Model file for the job. Use its own axes, mm. Give positions to 0.01 mm unless a question says otherwise; leave off trailing zeros. Order: outer loops, then holes, each group sorted by start corner. A loop starts at its lowest first (then second) coordinate and runs counter-clockwise, first axis right, second up. Notation, with made-up numbers: M 64,20.5 L 83,20.5 A33 cw 83,54.5 Z; hole C 8,-25 d1. An arc over 180 degrees is marked long. Return JSON: item names as keys, results as strings. Group by question number.
1. Slice it at A-A on z = 4. Give the number of separate pieces and of enclosed holes in the cut face, then the cut area to 3 significant figures.
2. Slice it at B-B on y = 16. List the corners of the cut face in (x, z) (3 decimals).
3. Slice it at D-D on y = -3. List the corners of the cut face in (x, z).
4. Wall check: probe 1 along X at (y, z) = (-8.5, 3.95); probe 2 along Y at (x, z) = (-1, 4.55); probe 3 along Z at (x, y) = (-2.5, 2). Give the ranges that are in metal, low to high. Write a range as [from, to].
from build123d import *

# Parameters (mm, degrees)
F0_W     = 40
F0_H     = 40
F1_DEPTH = 3.2
F2_R     = 2.425
F3_DEPTH = 1.6


with BuildPart() as f1:
    # F0 (on Top) → F1 (new body)
    with BuildSketch(Plane.XY):
        Rectangle(F0_W, F0_H)
    extrude(amount=F1_DEPTH)

    # F2 (on face) → F3 (join)
    with BuildSketch(Plane.XY.offset(3.2)):
        with Locations((-16, -16)):
            Circle(F2_R)
        with Locations((-16, -8)):
            Circle(F2_R)
        with Locations((-16, 0)):
            Circle(F2_R)
        with Locations((-16, 8)):
            Circle(F2_R)
        with Locations((-16, 16)):
            Circle(F2_R)
        with Locations((-8, -16)):
            Circle(F2_R)
        with Locations((-8, -8)):
            Circle(F2_R)
        with Locations((-8, 0)):
            Circle(F2_R)
        with Locations((-8, 8)):
            Circle(F2_R)
        with Locations((-8, 16)):
            Circle(F2_R)
        with Locations((0, -16)):
            Circle(F2_R)
        with Locations((0, -8)):
            Circle(F2_R)
        Circle(F2_R)
        with Locations((0, 8)):
            Circle(F2_R)
        with Locations((0, 16)):
            Circle(F2_R)
        with Locations((8, -16)):
            Circle(F2_R)
        with Locations((8, -8)):
            Circle(F2_R)
        with Locations((8, 0)):
            Circle(F2_R)
        with Locations((8, 8)):
            Circle(F2_R)
        with Locations((8, 16)):
            Circle(F2_R)
        with Locations((16, -16)):
            Circle(F2_R)
        with Locations((16, -8)):
            Circle(F2_R)
        with Locations((16, 0)):
            Circle(F2_R)
        with Locations((16, 8)):
            Circle(F2_R)
        with Locations((16, 16)):
            Circle(F2_R)
    extrude(amount=F3_DEPTH)


solid = f1.part
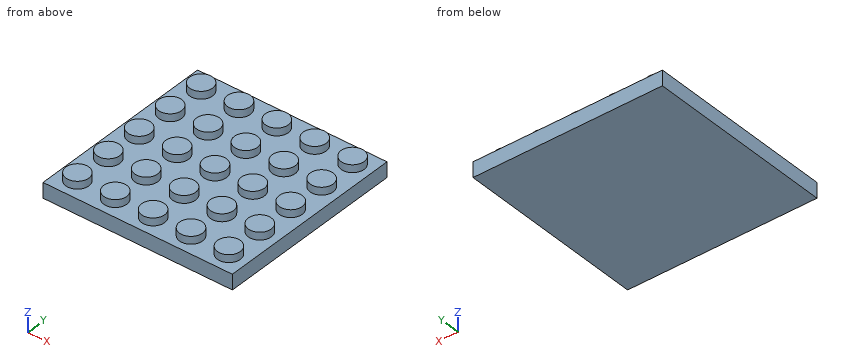
Result:
{
 "1": {"separate pieces": "25", "enclosed holes": "0", "area": "462 mm2"},
 "2": {"outline": "M -20,0 L 20,0 L 20,3.2 L 18.425,3.2 L 18.425,4.8 L 13.575,4.8 L 13.575,3.2 L 10.425,3.2 L 10.425,4.8 L 5.575,4.8 L 5.575,3.2 L 2.425,3.2 L 2.425,4.8 L -2.425,4.8 L -2.425,3.2 L -5.575,3.2 L -5.575,4.8 L -10.425,4.8 L -10.425,3.2 L -13.575,3.2 L -13.575,4.8 L -18.425,4.8 L -18.425,3.2 L -20,3.2 Z"},
 "3": {"outline": "M -20,0 L 20,0 L 20,3.2 L -20,3.2 Z"},
 "4": {"probe 1": "x = [-18.37, -13.63], [-10.37, -5.63], [-2.37, 2.37], [5.63, 10.37], [13.63, 18.37]", "probe 2": "y = [-18.21, -13.79], [-10.21, -5.79], [-2.21, 2.21], [5.79, 10.21], [13.79, 18.21]", "probe 3": "z = [0, 3.2]"}
}
